Could you check a few things on this drawing? It's one solid part, dimensions in mm from its lowest x, y, z. A direction names the side the tool comes from. Give positions to 0.01 mm unless a question says otherwise; leave off trailing zeros. Order: outer loops, then holes, each group sorted by start corner. A loop starts at its lowest first (then second) coordinate and runs counter-clockwise, first axis right, second up. Notation, with made-up numbers: (9, 76.25) - (35, 76.25) arc R13 cw to (35, 101.25) - close; hole circle Ø1 at (-11, 3.5). An arc over 180 degrees is marked (long way). Answer as CSV lines item,"result".
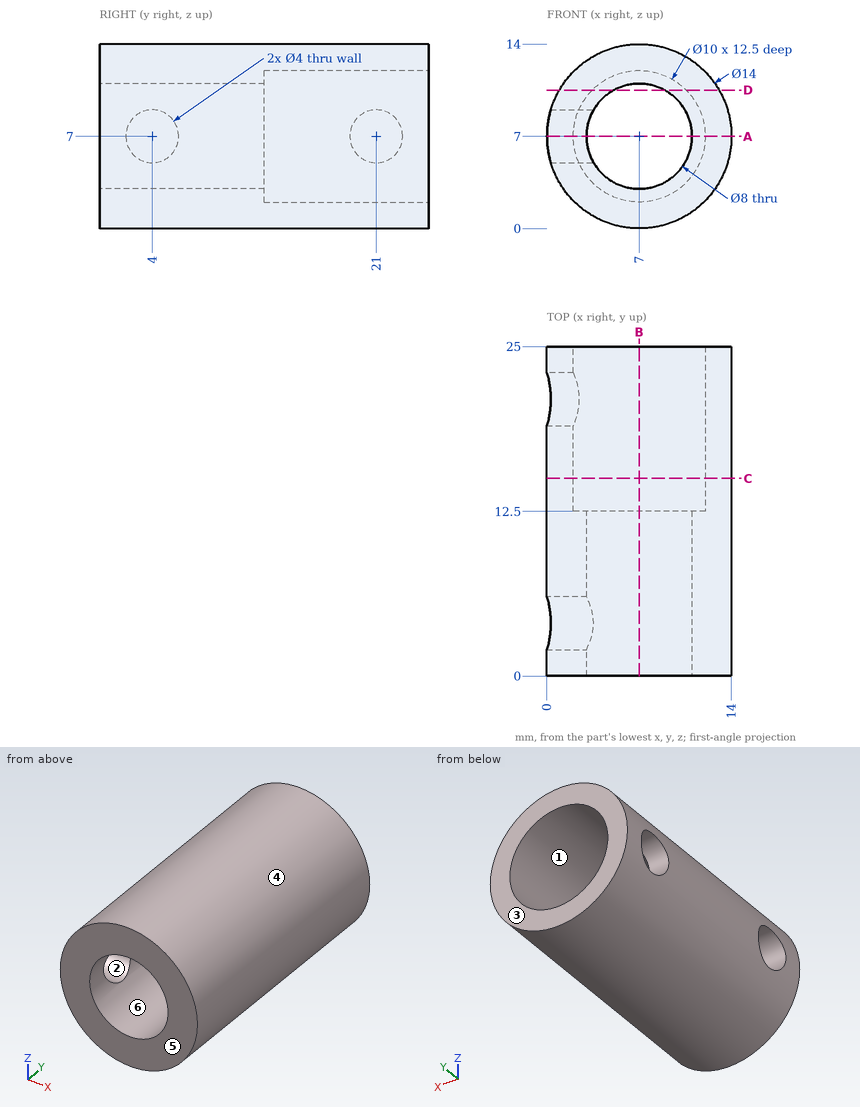
1) I want a section at B-B on x = 7. Write out the boundary of the cut face in (y, z), plus the area to 3 significant figures.
Answer block:
outline,"(0, 0) - (25, 0) - (25, 2) - (12.5, 2) - (12.5, 3) - (0, 3) - close; (0, 11) - (12.5, 11) - (12.5, 12) - (25, 12) - (25, 14) - (0, 14) - close"
area,"125 mm2"
2) If we mould it in two halves opening along X, with no side actions, what happens to the marked faces 4, 5 and 6? For each: +X half, -X half, draft (parallel to the pull), parting line (faces both ways), or undercut.
Answer block:
face 4,"parting line"
face 5,"draft"
face 6,"undercut"
3) I want a section at D-D on z = 10.5. Write out the boundary of the cut face in (x, y).
Answer block:
outline,"(0.94, 0) - (5.06, 0) - (5.06, 12.5) - (3.43, 12.5) - (3.43, 25) - (0.94, 25) - close; (8.94, 0) - (13.06, 0) - (13.06, 25) - (10.57, 25) - (10.57, 12.5) - (8.94, 12.5) - close"
4) I'm going to push flat-ended pins straight in: P1, Ø1.5, axis at y = 9, z = 11.5, coming from the -X side; P2, Ø6.5, axis at x = 7, z = 7, coming from the +Y side; P3, Ø5, axis at y = 17.5, z = 3, coming from the +X side; P4, Ø1.5, axis at x = 8, y = 21, coming from the -Z side. Where does each tip first touch, or does it pass through?
Answer block:
P1,"x = 1.09"
P2,"through"
P3,"x = 13.84"
P4,"z = 0"
5) I need wall thicknesses on line 1 along Z through (x, y) = (7, 17.5); line 2 along Z through (x, y) = (7, 6.75); line 3 along X through (y, z) = (17, 5.25). Which ranges of each line are inside material? Lowest first, please. Write a range as [from, to].
Answer block:
line 1,"[0, 2], [12, 14]"
line 2,"[0, 3], [11, 14]"
line 3,"[0.22, 2.32], [11.68, 13.78]"
6) Which directions (+Z, -Z, +X, -X, +Y, -Y) give clear straight access to the entire face, cutting with the end or side of a thin tool? Please do the marked faces 1, 2 and 3.
Answer block:
face 1,"+Y"
face 2,"-X"
face 3,"+Z, -Z, +X, -X, +Y"
7) I want a section at A-A on z = 7. Write out the boundary of the cut face in (x, y).
Answer block:
outline,"(0, 0) - (3, 0) - (3, 2) - (0, 2) - close; (0, 6) - (3, 6) - (3, 12.5) - (2, 12.5) - (2, 19) - (0, 19) - close; (0, 23) - (2, 23) - (2, 25) - (0, 25) - close; (11, 0) - (14, 0) - (14, 25) - (12, 25) - (12, 12.5) - (11, 12.5) - close"
8) I want a section at C-C on y = 15. Write out the boundary of the cut face in (x, z).
Answer block:
outline,"circle Ø14 at (7, 7); hole circle Ø10 at (7, 7)"
